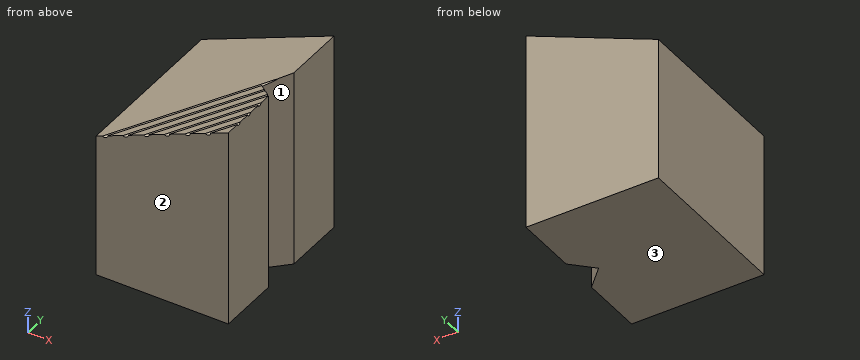
from build123d import *

# Parameters (mm, degrees)
F1_DEPTH = 25
F3_DEPTH = 30.001
F6_R     = 0.25
F7_DEPTH = 38.9529986152


with BuildPart() as f1:
    # F0 (on Front) → F1 (new body)
    with BuildSketch(Plane.XZ):
        Polygon((-20, 0), (0, 0), (0, 30), (-20, 21.7157287525), align=None)
    extrude(amount=F1_DEPTH)

    # F2 (on face) → F3 (cut, through all)
    with BuildSketch(Plane(origin=(0, 0, 0), x_dir=(1, 0, 0), z_dir=(0, 0, -1))):
        Polygon((0, 9.5), (0, 15.5), (-3, 12.5), align=None)
    extrude(amount=-F3_DEPTH, mode=Mode.SUBTRACT)

    # F6 (on line) → F7 (cut, through all)
    with BuildSketch(Plane(origin=(6.8564591979, 5.4885609135, 2.8400383896), x_dir=(-0.5493524956, 0.8040106793, -0.2275492542), z_dir=(0.7428090106, 0.5946148564, 0.3076815664))):
        with Locations((-14.9457916694, 27.7163859753)):
            Circle(F6_R)
        with Locations((-16.9457916694, 27.7163859753)):
            Circle(F6_R)
        with Locations((-18.9457916694, 27.7163859753)):
            Circle(F6_R)
        with Locations((-20.9457916694, 27.7163859753)):
            Circle(F6_R)
        with Locations((-22.9457916694, 27.7163859753)):
            Circle(F6_R)
        with Locations((-24.9457916694, 27.7163859753)):
            Circle(F6_R)
    extrude(amount=-F7_DEPTH, mode=Mode.SUBTRACT)


solid = f1.part
Here's how the part is built. I have some questions about the finished solid (model axes, mm). Face numbers are marked on the shaded views. Coordinates: 2 decimals unless noted, no trailing zeros. Loops run counter-clockwise (first coordinate to the right, second up) from the corner with the lowest first, then second, coordinate; pieces in that order, holes last.
1. I need wall thicknesses on L1, parallel to Z at x = -12, y = -3.5; L2, parallel to Z at x = -4.5, y = -7.25; L3, parallel to X at y = -10, z = 12. Which ranges of each line are inside material? Lowest first, please.
2. Imagine slicing it at A-A, the plane z = 6. Please give me the cut outline in (x, y).
3. For P1, Ø2, axis at y = -14, z = 19.5, coming from the +X side, with a flat end and sliding along its axis, tell me the tip position at first contact or that it passes through.
4. Imagine slicing it at B-B, the plane y = -9. Please give me the cut outline in (x, z).
5. If we mould it in two halves opening along Y, with no side actions, what happens to the marked faces 1, 2 and 3? For each: pulls with the +Y half, pulls with the -Y half, needs draft (parallel to the pull), parting line crosses it, or undercut.
Taken from the geometry:
1. L1: z = 0 to 25.03
1. L2: z = 0 to 28.14
1. L3: x = -20 to -0.5
2. outline: (-20, -25) - (0, -25) - (0, -15.5) - (-3, -12.5) - (0, -9.5) - (0, 0) - (-20, 0) - close
3. P1: stops at x = -0.5
4. outline: (-20, 0) - (0, 0) - (0, 30) - (-20, 21.72) - close
5. face 1: undercut
5. face 2: pulls with the -Y half
5. face 3: needs draft
